Here's how the part is built. I have some questions about the finished solid (model axes, mm). A direction names the side the tool comes from. Round coordinates to 2 decimals unless told otherwise and drop trailing zeros. Order: outer loops, then holes, each group sorted by start corner. A loop starts at its lowest first (then second) coordinate and runs counter-clockwise, first axis right, second up. Notation, with made-up numbers: (-23, 58.5) -> (12, 58.5) arc R18 cw to (12, 80.5) -> close; hole circle Ø6 at (14, 62). An arc over 180 degrees is marked (long way). Answer in a Markdown table with one row per item.
```python
from build123d import *

# Parameters (mm, degrees)
F3_DEPTH = 10


with BuildPart() as f3:
    # F2 (on Right) → F3 (new body)
    with BuildSketch(Plane.YZ):
        with BuildLine():
            Line((7.768028, 18), (7.768028, 37))
            Line((7.768028, 37), (7.368028, 37))
            Line((7.368028, 37), (5.768028, 35.093194))
            Line((5.768028, 35.093194), (5.768028, 33.676114))
            ThreePointArc((5.768028, 33.676114), (5.657029, 33.218209), (5.348673, 32.861957))
            ThreePointArc((5.348673, 32.861957), (3.567098, 32.144003), (1.654039, 32.316261))
            ThreePointArc((1.654039, 32.316261), (0.980832, 32.304735), (0.467528, 31.869007))
            Line((0.467528, 31.869007), (-10.456972, 12.947218))
            Line((-10.456972, 12.947218), (-9.574866, 12.437934))
            ThreePointArc((-9.574866, 12.437934), (-8.816046, 12.338033), (-8.20884, 12.803959))
            Line((-8.20884, 12.803959), (1.478715, 29.583296))
            ThreePointArc((1.478715, 29.583296), (1.883032, 29.970328), (2.431987, 30.079483))
            ThreePointArc((2.431987, 30.079483), (3.481519, 30.07755), (4.516067, 30.254275))
            ThreePointArc((4.516067, 30.254275), (5.379599, 30.077727), (5.768028, 29.286538))
            Line((5.768028, 29.286538), (5.768028, 17))
            ThreePointArc((5.768028, 17), (6.060921, 16.292893), (6.768028, 16))
            Line((6.768028, 16), (21.214821, 16))
            ThreePointArc((21.214821, 16), (21.921927, 16.292893), (22.214821, 17))
            Line((22.214821, 17), (22.214821, 18))
            Line((22.214821, 18), (7.768028, 18))
        make_face()
    extrude(amount=F3_DEPTH)


solid = f3.part
```
1. Please list where these lines run through material, in increasing order: line 1 along Z through (x, y) = (8, 12.5); line 2 along Y through (x, z) = (3.25, 34.5); line 3 along Y through (x, z) = (2.25, 24.25).
Numbers:
| item | result |
|---|---|
| line 1 | z = 16 to 18 |
| line 2 | y = 5.77 to 7.77 |
| line 3 | y = -3.93 to -1.6, 5.77 to 7.77 |
2. Suppose I cut it at C-C on y = 11.5. Write out the boundary of the cut face in (x, z), then the cut area to 3 significant figures.
Numbers:
| item | result |
|---|---|
| outline | (0, 16) -> (10, 16) -> (10, 18) -> (0, 18) -> close |
| area | 20.0 mm2 |
3. For pin 1 Ø5 at (x, z) = (4, 25.5) entering from +Y; pin 2 Ø6 at (x, z) = (4.5, 19) entering from +Y; pin 3 Ø5 at (x, y) = (3, 13) entering from +Z; pin 4 Ø1 at (x, y) = (4.5, 3.5) entering from +Z, each with a flat end and sliding along its axis, tell me the tip position at first contact or that it passes through.
Numbers:
| item | result |
|---|---|
| pin 1 | stops at y = 7.77 |
| pin 2 | stops at y = 22.21 |
| pin 3 | stops at z = 18 |
| pin 4 | stops at z = 32.23 |
4. For faces 5 (the face through (5, 7.768, 27)), 6 (the face through (5, 5.768, 34)), 7 (the face through (4.93, -3.43, 21.08)), 8 (the face through (5, 14, 16)), 9 (the face through (4.93, -10.022, 12.696)), which set-ups out of +Z, -Z, +X, -X, +Y, -Y let a thin tool reach every point of the face, with its end or its side?
Numbers:
| item | result |
|---|---|
| face 5 | +Z, +X, -X, +Y |
| face 6 | +Z, +X, -X, -Y |
| face 7 | -Z, +X, -X |
| face 8 | -Z, +X, -X, +Y |
| face 9 | -Z, +X, -X, -Y |
5. Suppose I cut it at A-A on z = 26.75. Write out the boundary of the cut face in (x, y).
Numbers:
| item | result |
|---|---|
| outline | (0, -2.49) -> (10, -2.49) -> (10, -0.16) -> (0, -0.16) -> close; (0, 5.77) -> (10, 5.77) -> (10, 7.77) -> (0, 7.77) -> close |
6. We'd pull the mould along Y, two halves only. Please class faces 1 (the face through (0, 6, 23)), 2 (the face through (4.9, 22.215, 17.5)), 3 (the face through (4.93, 3.594, 32.148)), 4 (the face through (4.93, 6.053, 16.301)): released by +Y, released by -Y, zero draft, split by the parting line, or undercut.
Numbers:
| item | result |
|---|---|
| face 1 | zero draft |
| face 2 | released by +Y |
| face 3 | undercut |
| face 4 | undercut |
7. Suppose I cut it at B-B on x = 6. Write out the boundary of the cut face in (y, z), then the cut area to 3 significant figures.
Numbers:
| item | result |
|---|---|
| outline | (-10.46, 12.95) -> (-9.57, 12.44) arc R1 ccw to (-8.21, 12.8) -> (1.48, 29.58) arc R1 cw to (2.43, 30.08) arc R6.14 ccw to (4.52, 30.25) arc R1 cw to (5.77, 29.29) -> (5.77, 17) arc R1 ccw to (6.77, 16) -> (21.21, 16) arc R1 ccw to (22.21, 17) -> (22.21, 18) -> (7.77, 18) -> (7.77, 37) -> (7.37, 37) -> (5.77, 35.09) -> (5.77, 33.68) arc R1 cw to (5.35, 32.86) arc R4.1 cw to (1.65, 32.32) arc R1 ccw to (0.47, 31.87) -> close |
| area | 123 mm2 |
8. Suppose I cut it at D-D on z = 17.5. Write out the boundary of the cut face in (x, y).
Numbers:
| item | result |
|---|---|
| outline | (0, -7.83) -> (10, -7.83) -> (10, -5.5) -> (0, -5.5) -> close; (0, 5.77) -> (10, 5.77) -> (10, 22.21) -> (0, 22.21) -> close |
